```python
from build123d import *

# Parameters (mm, degrees)
SKETCH1_W           = 60
SKETCH1_H           = 50
BOSS_EXTRUDE1_DEPTH = 50
SKETCH2_W           = 30
SKETCH2_H           = 10
CUT_EXTRUDE1_DEPTH  = 40
SKETCH3_W           = 30
SKETCH3_H           = 30
CUT_EXTRUDE2_DEPTH  = 30
SKETCH4_W           = 30
SKETCH4_H           = 10
BOSS_EXTRUDE2_DEPTH = 7
SKETCH5_W           = 30
SKETCH5_H           = 30
BOSS_EXTRUDE3_DEPTH = 12
CUT_EXTRUDE6_DEPTH  = 10
CUT_EXTRUDE7_DEPTH  = 20
CUT_EXTRUDE8_DEPTH  = 52
SKETCH13_W          = 30
SKETCH13_H          = 30
BOSS_EXTRUDE4_DEPTH = 1.5


with BuildPart() as part:
    # Sketch1 → Boss-Extrude1 (new body)
    with BuildSketch(Plane.XY):
        with Locations((30, 25)):
            Rectangle(SKETCH1_W, SKETCH1_H)
    extrude(amount=BOSS_EXTRUDE1_DEPTH)

    # Sketch2 → Cut-Extrude1 (cut)
    with BuildSketch(Plane.XY.offset(50)):
        with Locations((15, 45)):
            Rectangle(SKETCH2_W, SKETCH2_H)
    extrude(amount=-CUT_EXTRUDE1_DEPTH, mode=Mode.SUBTRACT)

    # Sketch3 → Cut-Extrude2 (cut)
    with BuildSketch(Plane.XY.offset(50)):
        with Locations((45, 35)):
            Rectangle(SKETCH3_W, SKETCH3_H)
    extrude(amount=-CUT_EXTRUDE2_DEPTH, mode=Mode.SUBTRACT)

    # Sketch4 → Boss-Extrude2 (add)
    with BuildSketch(Plane.XY.offset(10)):
        with Locations((15, 45)):
            Rectangle(SKETCH4_W, SKETCH4_H)
    extrude(amount=BOSS_EXTRUDE2_DEPTH)

    # Sketch5 → Boss-Extrude3 (add)
    with BuildSketch(Plane.XY.offset(20)):
        with Locations((45, 35)):
            Rectangle(SKETCH5_W, SKETCH5_H)
    extrude(amount=BOSS_EXTRUDE3_DEPTH)

    # Sketch10 → Cut-Extrude6 (cut)
    with BuildSketch(Plane(origin=(0, 0, 0), x_dir=(0, 0, -1), z_dir=(1, 0, 0))):
        Polygon((-17, 40), (-50, 0), (-50, 40), align=None)
    extrude(amount=CUT_EXTRUDE6_DEPTH, mode=Mode.SUBTRACT)

    # Sketch11 → Cut-Extrude7 (cut)
    with BuildSketch(Plane.ZY.offset(-10)):
        Polygon((17, 40), (50, 40), (50, 0), align=None)
    extrude(amount=-CUT_EXTRUDE7_DEPTH, mode=Mode.SUBTRACT)

    # Sketch12 → Cut-Extrude8 (cut)
    with BuildSketch(Plane.ZY.offset(-30)):
        Polygon((33.5, 20), (50, 0), (50, 20), align=None)
    extrude(amount=-CUT_EXTRUDE8_DEPTH, mode=Mode.SUBTRACT)

    # Sketch13 → Boss-Extrude4 (add)
    with BuildSketch(Plane.XY.offset(32)):
        with Locations((45, 35)):
            Rectangle(SKETCH13_W, SKETCH13_H)
    extrude(amount=BOSS_EXTRUDE4_DEPTH)


solid = part.part
```
Model file for the job. Use its own axes, mm. A direction names the side the tool comes from. Coordinates: 2 decimals unless noted, no trailing zeros. Write each loop counter-clockwise with the first axis right and the second up, starting at its lowest first coordinate (ties: lowest second). Pieces come first, ordered by that corner, then holes. Notation, with made-up numbers: (31, -37.5) - (52, -37.5) arc R11 ccw to (52, -31.5) - close; hole circle Ø7 at (-6.75, 9.5). An arc over 180 degrees is marked (long way). One line per item, written item: value. Start each with the question number.
1. Tool access for faces 1 (the flat face through (30, 38, 27)), 2 (the flat face through (30, 25, 0)), 3 (the flat face through (45, 35, 33.5)): list every direction of +Z, -Z, +X, -X, +Y, -Y with a clear straight run to the whole face (end or side of a thin tool).
2. Probe line 1 (X direction, y = 42, z = 23); line 2 (Z direction, x = 40, y = 28); line 3 (Z direction, x = 28, y = 43.5). List the from-to ranges inside material, lowest first. Write a range as from..to.
3. Slice it at C-C (z = 24). Write the cut outline in (x, y), plus the area to 3 significant figures.
4. Slice it at D-D (x = 8). Write the cut outline in (y, z), plus the area to 3 significant figures.
5. Slice it at B-B (x = 52). Write the cut outline in (y, z).
6. Slice it at A-A (y = 30). Write the cut outline in (x, z), plus the area to 3 significant figures.
7. Flat gauge pins, fed straight in: pin 1 (3 mm diameter, centred on x = 18.5, y = 43.5, fed in from +Z); pin 2 (24 mm diameter, centred on x = 43, y = 29.5, fed in from +Z); pin 3 (1.5 mm diameter, centred on x = 47, y = 35, fed in from +Z). Where does each tip first touch, or does it go through?
Answers below:
1. face 1: +Z, -X, +Y
1. face 2: -Z, +X, -X, +Y, -Y
1. face 3: +Z, +X, -X, +Y
2. line 1: x = 30..60
2. line 2: z = 0..33.5
2. line 3: z = 0..17
3. outline: (0, 0) - (60, 0) - (60, 50) - (30, 50) - (30, 31.52) - (0, 31.52) - close
3. area: 2,450 mm^2
4. outline: (0, 0) - (50, 0) - (50, 17) - (40, 17) - (0, 50) - close
4. area: 1,510 mm^2
5. outline: (0, 0) - (50, 0) - (50, 33.5) - (20, 33.5) - (0, 50) - close
6. outline: (0, 0) - (60, 0) - (60, 33.5) - (30, 33.5) - (30, 25.25) - (0, 25.25) - close
6. area: 1,760 mm^2
7. pin 1: stops at z = 17
7. pin 2: stops at z = 35.56
7. pin 3: stops at z = 33.5
